Autodesk Inventor part; units mm, degrees
ref_plane "YZ Plane" through (0, 0, 0) normal (1, 0, 0) x (0, 1, 0)
ref_plane "XZ Plane" through (0, 0, 0) normal (0, 1, 0) x (-1, 0, 0)
ref_plane "XY Plane" through (0, 0, 0) normal (0, 0, 1) x (1, 0, 0)
sketch "Sketch1" plane through (0, 0, 0) normal (0, 1, 0) x (-1, 0, 0)
  line L0 (349.8743, 0) -> (258.4057, -158.4282)
  line L1 (174.9371, -303) -> (-174.9371, -303)
  line L2 (-174.9371, -303) -> (-349.8743, 0)
  line L3 (-349.8743, 0) -> (-174.9371, 303)
  line L4 (-174.9371, 303) -> (174.9371, 303)
  line L5 (258.4057, 158.4282) -> (349.8743, 0)
  line L6 (0, 0) -> (-8, 0)
  line L7 (-8, 0) -> (-8, -303)
  line L8 (-8, -303) -> (8, -303)
  line L9 (8, -303) -> (8, 0)
  line L10 (8, 0) -> (-8, 0)
  circle A0 centre (0, 0) radius 2.5
  line L11 (258.4057, 158.4282) -> (-4, 6.9282)
  line L12 (4, -6.9282) -> (266.4057, 144.5718)
  line L13 (-4, 6.9282) -> (4, -6.9282)
  line L14 (-266.4057, 144.5718) -> (-4, -6.9282)
  line L15 (4, 6.9282) -> (-258.4057, 158.4282)
  line L16 (-4, -6.9282) -> (4, 6.9282)
  line L17 (8, -4.6188) -> (8, -151.5)
  line L18 (8, -151.5) -> (-8, -151.5)
  line L19 (-8, -151.5) -> (-8, -303)
  line L20 (-8, -4.6188) -> (-4, -6.9282)
  line L21 (4, -6.9282) -> (-4, -6.9282)
  line L22 (-266.4057, 144.5718) -> (-258.4057, 158.4282)
  line L23 (-127.2028, 82.6782) -> (-135.2028, 68.8218)
  line L24 (-135.2028, 68.8218) -> (-8, -4.6188)
  line L25 (-266.4057, 144.5718) -> (-349.8743, 0)
  line L26 (-174.9371, -303) -> (-349.8743, 0)
  line L27 (-174.9371, -303) -> (-8, -303)
  line L28 (0, 9.2376) -> (8, 0)
  dimension "d0" = 303
  dimension "d1" = 303
  dimension "d2" = 8
  dimension "d3" = 16
  dimension "d4" = 5
  dimension "d7" = 360
extrude "Extrusion1" add sketch "Sketch1" along normal blind 3 contours L1 L7 L18 L9 | L1 L2 L3 L14 L7 | L18 L7 L14 L21 L12 L9 | L12 L13 A0 L10 L9 | L14 L23 L15 L11 L13 A0 L6 L7 | L7 L6 A0 L16 L14 | L10 A0 L16 L28 | L21 L16 A0 L13 | L3 L15 L23 L14 | A0 L13 L10 | L10 L16 A0 | L28 L15 L16 | L16 A0 L13 L11 L28 | A0 L16 L13 | A0 L13 L6 | L6 L16 A0 | L13 A0 L16
sketch "Sketch2" plane through (0, 3, 0) normal (0, 1, 0) x (1, 0, 0)
  line L0 (-8, 303) -> (-8, 0)
  line L1 (-8, 0) -> (-8, 151.5)
  line L2 (-8, 151.5) -> (8, 151.5)
  line L3 (8, 151.5) -> (8, 0)
  line L4 (8, 0) -> (-8, 0)
  line L5 (0, -9.2376) -> (258.4057, -158.4282)
  line L6 (258.4057, -158.4282) -> (126.3368, -82.1782)
  line L7 (126.3368, -82.1782) -> (134.8368, -67.4558)
  line L8 (134.8368, -67.4558) -> (266.9057, -143.7058)
  line L9 (266.9057, -143.7058) -> (258.4057, -158.4282)
  point P0 (0, 0)
  dimension "d11" = 151.5
  dimension "d12" = 16
  dimension "d13" = 152.5
  dimension "d14" = 17
extrude "Extrusion2" cut sketch "Sketch2" against normal blind 3
sketch "Sketch3" plane through (0, 3, 0) normal (0, 1, 0) x (1, 0, 0)
  line L0 (174.9371, 303) -> (-8, 303)
  line L1 (174.9371, 303) -> (149.9371, 303)
  line L2 (149.9371, 303) -> (149.9371, 297)
  line L3 (149.9371, 297) -> (174.9371, 297)
  line L4 (174.9371, 297) -> (174.9371, 303)
  line L5 (349.8743, 0) -> (174.9371, 303)
  line L6 (174.9371, 303) -> (187.4371, 281.3494)
  line L7 (187.4371, 281.3494) -> (182.241, 278.3494)
  line L8 (182.241, 278.3494) -> (169.741, 300)
  line L9 (169.741, 300) -> (174.9371, 303)
  line L10 (349.8743, 0) -> (337.3743, 21.6506)
  line L11 (337.3743, 21.6506) -> (332.1781, 18.6506)
  line L12 (332.1781, 18.6506) -> (344.6781, -3)
  line L13 (344.6781, -3) -> (349.8743, 0)
  line L14 (349.8743, 0) -> (337.3743, -21.6506)
  line L15 (337.3743, -21.6506) -> (332.1781, -18.6506)
  line L16 (332.1781, -18.6506) -> (344.6781, 3)
  line L17 (344.6781, 3) -> (349.8743, 0)
  line L18 (349.8743, 0) -> (266.9057, -143.7058)
  line L19 (349.8743, 0) -> (374.8743, 0) construction
  point P0 (0, 0)
  dimension "d17" = 25
  dimension "d18" = 6
  dimension "d19" = 25
  dimension "d20" = 6
  dimension "d21" = 25
  dimension "d22" = 6
  dimension "d23" = 25
  dimension "d24" = 120
  dimension "d25" = 6
extrude "Extrusion3" cut sketch "Sketch3" against normal blind 3
sketch "Sketch4" plane through (0, 3, 0) normal (0, 1, 0) x (1, 0, 0)
  line L0 (-55.0368, 49.6734) -> (70.5368, -22.8266)
  line L1 (70.5368, -22.8266) -> (55.0368, -49.6734)
  line L2 (55.0368, -49.6734) -> (-70.5368, 22.8266)
  line L3 (-70.5368, 22.8266) -> (-55.0368, 49.6734)
  line L4 (-55.0368, 49.6734) -> (55.0368, -49.6734) construction
  line L5 (70.5368, -22.8266) -> (-70.5368, 22.8266) construction
  line L6 (-55.0368, 49.6734) -> (89.9632, 49.6734) construction
  line L7 (-15.5, -72.5) -> (-15.5, 72.5)
  line L8 (-15.5, 72.5) -> (15.5, 72.5)
  line L9 (15.5, 72.5) -> (15.5, -72.5)
  line L10 (15.5, -72.5) -> (-15.5, -72.5)
  line L11 (-15.5, -72.5) -> (15.5, 72.5) construction
  line L12 (-15.5, 72.5) -> (15.5, -72.5) construction
  line L13 (-8, 0) -> (8, 0)
  line L14 (-15.5, -72.5) -> (129.5, -72.5) construction
  point P0 (0, 0)
  dimension "d28" = 145
  dimension "d29" = 30
  dimension "d30" = 31
  dimension "d31" = 145
  dimension "d32" = 90
  dimension "d33" = 31
extrude "Extrusion4" cut sketch "Sketch4" against normal blind 3
sketch "Sketch5" plane through (0, 3, 0) normal (0, 1, 0) x (1, 0, 0)
  line L0 (-1, 151.5) -> (-1, 191.5)
  circle A0 centre (-1, 191.5) radius 2.75
  circle A1 centre (-1, 231.5) radius 2.75
  circle A2 centre (-1, 271.5) radius 2.75
  circle A3 centre (0, 0) radius 0.5
  line L1 (126.3368, -82.1782) -> (134.8368, -67.4558)
  line L2 (126.3368, -82.1782) -> (129.3368, -76.9821)
  line L3 (129.3368, -76.9821) -> (103.3561, -61.9821)
  line L4 (103.3561, -61.9821) -> (77.3753, -46.9821)
  circle A4 centre (103.3561, -61.9821) radius 2.75
  circle A5 centre (77.3753, -46.9821) radius 2.75
  line L5 (-8, 303) -> (-8, 151.5)
  dimension "d36" = 40
  dimension "d37" = 5.5
  dimension "d40" = 40
  dimension "d45" = 1
  dimension "d46" = 6
  dimension "d47" = 30
  dimension "d48" = 30
  dimension "d49" = 5.5
  dimension "d50" = 5.5
  dimension "d53" = 7
extrude "Extrusion5" cut sketch "Sketch5" against normal blind 3 contours A0 | A1 | A2 | A4 L4 L3 | A5 | L3 L4 A4
sketch "Sketch6" plane through (0, 3, 0) normal (0, 1, 0) x (1, 0, 0)
  line L0 (-8, 303) -> (-8, 151.5)
  line L1 (-8, 303) -> (344, 303)
  line L2 (344, 303) -> (344, -147)
  line L3 (344, -147) -> (-8, -147)
  line L4 (-8, -147) -> (-8, 303)
  point P0 (0, 0)
  dimension "d54" = 352
  dimension "d55" = 450
sketch "Sketch7" plane through (0, 3, 0) normal (0, 1, 0) x (1, 0, 0)
  line L0 (0, 0) -> (86.6025, 50)
  line L1 (0, 0) -> (100, 0) construction
  line L2 (86.6025, 50) -> (91.8525, 40.9067)
  circle A0 centre (91.8525, 40.9067) radius 1.1
  line L3 (86.6025, 50) -> (89.2006, 51.5)
  line L4 (86.6025, 50) -> (89.6025, 50) construction
  circle A1 centre (81.3525, 59.0933) radius 1.1
  circle A2 centre (102.6779, 47.1567) radius 1.1
  circle A3 centre (92.1779, 65.3433) radius 1.1
  dimension "d56" = 100
  dimension "d57" = 30
  dimension "d58" = 10.5
  dimension "d59" = 90
  dimension "d60" = 2.2
  dimension "d61" = 3
  dimension "d62" = 30
  dimension "d65" = 21
  dimension "d68" = 12.5
extrude "Extrusion6" cut sketch "Sketch7" against normal blind 5
properties part number "Acrylic_bottom_camera"
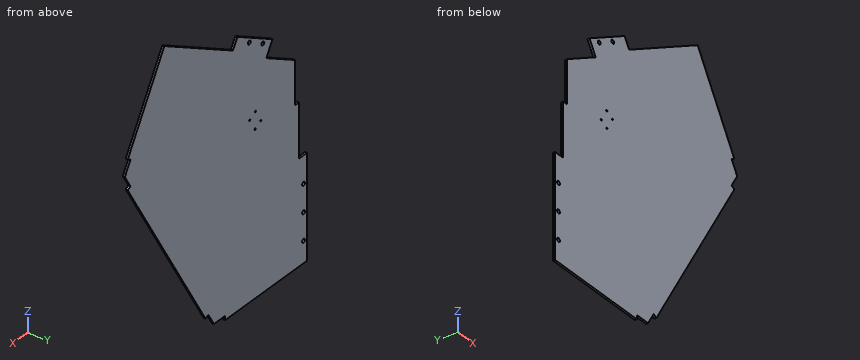
Here's how the part is built. I have some questions about the finished solid (model axes, mm). Round coordinates to 2 decimals unless told otherwise and drop trailing zeros. Loops run counter-clockwise (first coordinate to the right, second up) from the corner with the lowest first, then second, coordinate; pieces in that order, holes last.
1. If we section it at A-A on y = 2.25: Count the separate pieces of the cut face and the enclosed holes in it, plus the area to 3 significant figures.
Answer list:
separate pieces: 1
enclosed holes: 9
area: 103,000 mm2
2. If we section it at C-C on x = 220: Write out the boundary of the cut face in (y, z), plus the area to 3 significant figures.
Answer list:
outline: (0, -224.95) - (3, -224.95) - (3, 116.62) - (0, 116.62) - close
area: 1,020 mm2
3. For P1, Ø2, axis at x = 92.18, z = -65.34, coming from the +Y side; P2, Ø0.9, axis at x = 11.5, y = 2, coming from the +Z side; P3, Ø0.9, axis at y = 1.5, z = -100.5, coming from the -X side; P4, Ø1.5, axis at y = 1, z = -300, coming from the +X side, each with a flat end and sliding along its axis, tell me the tip position at first contact or that it passes through.
Answer list:
P1: passes through
P2: stops at z = -72.5
P3: stops at x = 8
P4: stops at x = 149.94
4. If I drill on line 1 along Z through (x, y) = (-1, 2.2); line 2 along X through (y, z) = (1.7, -191.5); line 3 along X through (y, z) = (0.6, -48), over which ranges is the centre line in solid material (lowest first)?
Answer list:
line 1: z = -303 to -274.25, -268.75 to -234.25, -228.75 to -194.25, -188.75 to -151.5
line 2: x = -8 to -3.75, 1.75 to 239.31
line 3: x = 15.5 to 101.97, 103.38 to 322.16
5. If we section it at B-B on z = -252: Write out the boundary of the cut face in (x, y).
Answer list:
outline: (-8, 0) - (204.38, 0) - (204.38, 3) - (-8, 3) - close
